from build123d import *

# Parameters (mm, degrees)
F1_DEPTH = 3
F3_DEPTH = 1
F4_R     = 1.5
F5_DEPTH = 25


with BuildPart() as f1:
    # F0 (on Top) → F1 (new body)
    with BuildSketch(Plane.XY):
        with BuildLine():
            Line((14.9, 19), (-15, 19))
            ThreePointArc((-15, 19), (-17.828427, 17.828427), (-19, 15))
            Line((-19, 15), (-19, -14.9))
            ThreePointArc((-19, -14.9), (-17.828427, -17.728427), (-15, -18.9))
            Line((-15, -18.9), (14.9, -18.9))
            ThreePointArc((14.9, -18.9), (17.728427, -17.728427), (18.9, -14.9))
            Line((18.9, -14.9), (18.9, 15))
            ThreePointArc((18.9, 15), (17.728427, 17.828427), (14.9, 19))
        make_face()
    extrude(amount=F1_DEPTH)

    # F2 (on face) → F3 (cut)
    with BuildSketch(Plane.XY.offset(3)):
        with BuildLine():
            Line((-14, 6), (-19, 6))
            Line((-19, 6), (-19, 0))
            Line((-19, 0), (-14, 0))
            ThreePointArc((-14, 0), (-11.87868, 0.87868), (-11, 3))
            ThreePointArc((-11, 3), (-11.87868, 5.12132), (-14, 6))
        make_face()
        with BuildLine():
            Line((18.9, 19), (10.9, 19))
            Line((10.9, 19), (10.9, 14))
            ThreePointArc((10.9, 14), (11.77868, 11.87868), (13.9, 11))
            Line((13.9, 11), (18.9, 11))
            Line((18.9, 11), (18.9, 19))
        make_face()
        with BuildLine():
            Line((-14, -10.9), (-19, -10.9))
            Line((-19, -10.9), (-19, -18.9))
            Line((-19, -18.9), (-11, -18.9))
            Line((-11, -18.9), (-11, -13.9))
            ThreePointArc((-11, -13.9), (-11.87868, -11.77868), (-14, -10.9))
        make_face()
        with BuildLine():
            Line((18.9, -18.9), (18.9, -10.9))
            Line((18.9, -10.9), (13.9, -10.9))
            ThreePointArc((13.9, -10.9), (11.77868, -11.77868), (10.9, -13.9))
            Line((10.9, -13.9), (10.9, -18.9))
            Line((10.9, -18.9), (18.9, -18.9))
        make_face()
    extrude(amount=-F3_DEPTH, mode=Mode.SUBTRACT)

    # F4 (on face) → F5 (cut)
    with BuildSketch(Plane.XY.offset(2)):
        with Locations((-15.75, 3)):
            Circle(F4_R)
        with Locations((15.75, 15)):
            Circle(F4_R)
        with Locations((15.75, -15)):
            Circle(F4_R)
        with Locations((-15.75, -15)):
            Circle(F4_R)
    extrude(amount=-F5_DEPTH, mode=Mode.SUBTRACT)


solid = f1.part
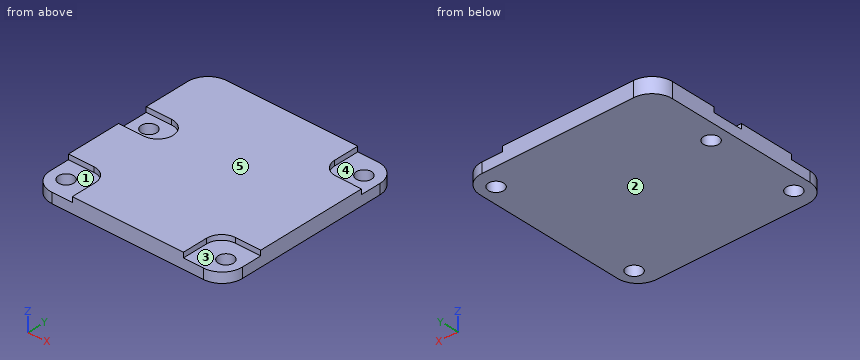
Verification items for the finished model (mm, model axes). Face numbers are marked on the shaded views. A direction names the side the tool comes from. Coordinates: 2 decimals unless noted, no trailing zeros. Loops run counter-clockwise (first coordinate to the right, second up) from the corner with the lowest first, then second, coordinate; pieces in that order, holes last. Notation, with made-up numbers: (13, -29) -> (45, -29) arc R16 ccw to (45, -22) -> close; hole circle Ø11 at (-23, 9). An arc over 180 degrees is marked (long way). Answer as a JSON object with one key per item and string values. Group by question number.
Item 1: Tool access check on the marked faces 1, 2, 3, 4 and 5. Record the directions out of +Z, -Z, +X, -X, +Y, -Y that give a thin tool (end or side, any length) a straight path to the whole face; none if there is none.
Item 2: Scan lines: probe 1 along Y at (x, z) = (14.5, 0.5); probe 2 along Y at (x, z) = (-15.75, 0.6); probe 3 along X at (y, z) = (-14.5, 1.55). Record each from-to range of solid material in increasing order.
Item 3: Sectioned sample at C-C on z = 0.8. Record the boundary of the cut face in (x, y).
Item 4: Sectioned sample at A-A on y = 16. Record the boundary of the cut face in (x, z), plus the area to 3 significant figures.
Item 5: Depth check by flat-ended pin: pin 1 (3 mm diameter, centred on x = -13, y = 3.5, fed in from +Z); pin 2 (0.8 mm diameter, centred on y = -15.5, z = 2.5, fed in from -X); pin 3 (0.8 mm diameter, centred on x = -16.5, z = 2.5, fed in from -Y). Enter the tip coordinate at first touch or a pass-through.
Item 6: Sectioned sample at D-D on y = 12. Record the boundary of the cut face in (x, z), plus the area to 3 significant figures.
Item 7: Sectioned sample at B-B on x = -15.75. Record the boundary of the cut face in (y, z).
Evaluation:
{
 "1": {"face 1": "+Z, -X, -Y", "face 2": "-Z, +X, -X, +Y, -Y", "face 3": "+Z, +X, -Y", "face 4": "+Z, +X, +Y", "face 5": "+Z, +X, -X, +Y, -Y"},
 "2": {"probe 1": "y = -18.9 to -15.83, -14.17 to 14.17, 15.83 to 19", "probe 2": "y = -18.83 to -16.5, -13.5 to 1.5, 4.5 to 18.93", "probe 3": "x = -19 to -17.16, -14.34 to 14.34, 17.16 to 18.9"},
 "3": {"outline": "(-19, -14.9) arc R4 ccw to (-15, -18.9) -> (14.9, -18.9) arc R4 ccw to (18.9, -14.9) -> (18.9, 15) arc R4 ccw to (14.9, 19) -> (-15, 19) arc R4 ccw to (-19, 15) -> close; hole circle Ø3 at (-15.75, -15); hole circle Ø3 at (-15.75, 3); hole circle Ø3 at (15.75, -15); hole circle Ø3 at (15.75, 15)"},
 "4": {"outline": "(-18.87, 0) -> (14.63, 0) -> (14.63, 2) -> (10.9, 2) -> (10.9, 3) -> (-18.87, 3) -> close; (16.87, 0) -> (18.77, 0) -> (18.77, 2) -> (16.87, 2) -> close", "area": "101 mm²"},
 "5": {"pin 1": "stops at z = 2", "pin 2": "stops at x = -11", "pin 3": "stops at y = -10.9"},
 "6": {"outline": "(-19, 0) -> (18.9, 0) -> (18.9, 2) -> (11.66, 2) -> (11.66, 3) -> (-19, 3) -> close", "area": "106 mm²"},
 "7": {"outline": "(-18.83, 0) -> (-16.5, 0) -> (-16.5, 2) -> (-18.83, 2) -> close; (-13.5, 0) -> (1.5, 0) -> (1.5, 2) -> (0, 2) -> (0, 3) -> (-10.9, 3) -> (-10.9, 2) -> (-13.5, 2) -> close; (4.5, 0) -> (18.93, 0) -> (18.93, 3) -> (6, 3) -> (6, 2) -> (4.5, 2) -> close"}
}
